Geometry check sheet. Reference: the model listing, model coordinates, mm. Coordinates: 2 decimals unless noted, no trailing zeros. Loops run counter-clockwise (first coordinate to the right, second up) from the corner with the lowest first, then second, coordinate; pieces in that order, holes last. Notation, with made-up numbers: (75, -10.75) -> (134, -10.75) arc R21 cw to (134, -6.75) -> close; hole circle Ø7 at (50.5, 44.5). An arc over 180 degrees is marked (long way). Answer as a JSON object with one key per item and string values.
from build123d import *

# Parameters (mm, degrees)
SKETCH_R  = 3
PAD_DEPTH = 10


with BuildPart() as part:
    # Sketch → Pad (new body)
    with BuildSketch(Plane.XY):
        with BuildLine():
            Line((0, 0), (80, 0))
            Line((80, 0), (80, 36))
            ThreePointArc((80, 36), (69.46807, 47.90986), (56.359205, 38.914086))
            ThreePointArc((22.759205, 35.314086), (40.815609, 25.387649), (56.359205, 38.914086))
            ThreePointArc((22.759205, 35.314086), (9.27149, 41.685685), (0, 30))
            Line((0, 30), (0, 0))
        make_face()
        with Locations((68, 36)):
            Circle(SKETCH_R, mode=Mode.SUBTRACT)
        with Locations((12, 30)):
            Circle(SKETCH_R, mode=Mode.SUBTRACT)
    extrude(amount=PAD_DEPTH)


solid = part.part
1. Depth check by flat-ended pin: P1, Ø5, axis at x = 12, y = 30, coming from the +Z side; P2, Ø6, axis at x = 29.5, z = 5, coming from the +Y side. Enter the tip coordinate at first touch or a pass-through.
Evaluation:
{"P1": "passes through", "P2": "stops at y = 30.24"}
2. Section check C-C, the plane x = 12. Record the boundary of the cut face in (y, z).
Evaluation:
{"outline": "(0, 0) -> (27, 0) -> (27, 10) -> (0, 10) -> close; (33, 0) -> (42, 0) -> (42, 10) -> (33, 10) -> close"}
3. Section check B-B, the plane z = 4.5. Record the boundary of the cut face in (x, y), then the cut area to 3 significant figures.
Evaluation:
{"outline": "(0, 0) -> (80, 0) -> (80, 36) arc R12 ccw to (56.36, 38.91) arc R18 cw to (22.76, 35.31) arc R12 ccw to (0, 30) -> close; hole circle Ø6 at (12, 30); hole circle Ø6 at (68, 36)", "area": "2,880 mm^2"}
4. Thickness scan on probe 1 along Y at (x, z) = (12, 2.75); probe 2 along X at (y, z) = (30.5, 7.5); probe 3 along X at (y, z) = (36.5, 7.5). Record the ranges inside material, lowest first. Write a range as from..to.
Evaluation:
{"probe 1": "y = 0..27, 33..42", "probe 2": "x = 0.01..9.04, 14.96..26.23, 51.57..80", "probe 3": "x = 1.91..22.09, 55.57..65.04, 70.96..79.99"}
5. Mould release check, pull along X, two halves, no side actions. Record for faces 1 (the face through (39, 19, 10)), 2 (the face through (9.79, 32.03, 4.93)), 3 (the face through (0, 15, 5)): released by +X, released by -X, zero draft, split by the parting line, or undercut.
Evaluation:
{"face 1": "zero draft", "face 2": "undercut", "face 3": "released by -X"}
6. Section check D-D, the plane x = 40.5. Record the boundary of the cut face in (y, z), then the cut area to 3 significant figures.
Evaluation:
{"outline": "(0, 0) -> (25.36, 0) -> (25.36, 10) -> (0, 10) -> close", "area": "254 mm^2"}
7. Section check A-A, the plane x = 68. Record the boundary of the cut face in (y, z), then the cut area to 3 significant figures.
Evaluation:
{"outline": "(0, 0) -> (33, 0) -> (33, 10) -> (0, 10) -> close; (39, 0) -> (48, 0) -> (48, 10) -> (39, 10) -> close", "area": "420 mm^2"}
